The listing builds one solid part. Answer for the finished solid, in the listing's coordinates (mm). A direction names the side the tool comes from. Coordinates: 2 decimals unless noted, no trailing zeros. Order: outer loops, then holes, each group sorted by start corner. A loop starts at its lowest first (then second) coordinate and runs counter-clockwise, first axis right, second up. Notation, with made-up numbers: (-6.5, -7) -> (26.5, -7) arc R9 cw to (26.5, 7) -> close; hole circle Ø1 at (83, 62). An arc over 180 degrees is marked (long way). Return JSON: item names as keys, results as strings.
from build123d import *

# Parameters (mm, degrees)
SKETCH2_W                     = 34
SKETCH2_H                     = 34
BOSS_EXTRUDE_MAIN_DEPTH       = 4.5
SKETCH9_W                     = 14
SKETCH9_H                     = 12.7
CUT_USBC_HOLE_DEPTH           = 5.5
SKETCH10_W                    = 22.5
SKETCH10_H                    = 3.4
CUT_FOURPIN_NOTCH_DEPTH       = 15.7
SKETCH11_R                    = 2
BOSS_EXTRUDE_PEGSPACERS_DEPTH = 2.5
F_2_0MM_HOLES_FOR_PEGS_D      = 1.7
F_2_0MM_HOLES_FOR_PEGS_DEPTH  = 4
F_2_0MM_HOLES_FOR_PEGS_TIP    = 0.510731526
SKETCH15_R                    = 15.4
SKETCH15_R_2                  = 12
CUT_SM1_DEPTH                 = 1
SKETCH18_W                    = 1.4
SKETCH18_H                    = 4.1
CUT_HEXNUTRIGHT_DEPTH         = 1
CUT_HEXNUTRIGHT_DEPTH_BACK    = 6.75
SKETCH19_W                    = 1.4
SKETCH19_H                    = 4.1
CUT_HEXNUTLEFT_DEPTH          = 6.75
SKETCH20_W                    = 18
SKETCH20_H                    = 34
CUT_EXTRUDE2_DEPTH            = 1.5
SKETCH21_W                    = 34
SKETCH21_H                    = 18
CUT_EXTRUDE3_DEPTH            = 1.5
SKETCH22_W                    = 13
SKETCH22_H                    = 10
BOSS_EXTRUDE1_DEPTH           = 10.5
CUT_EXTRUDE4_DEPTH            = 15
SKETCH25_W                    = 2
SKETCH25_H                    = 10
CUT_EXTRUDE5_DEPTH            = 15
SKETCH22_2_W                  = 13
SKETCH22_2_H                  = 10
BOSS_EXTRUDE2_DEPTH           = 1
CUT_EXTRUDE6_DEPTH            = 2
FILLET5_R                     = 3
FILLET4_R                     = 3
FILLET3_R                     = 3
FILLET2_R                     = 3
FILLET7_R                     = 2
FILLET8_R                     = 2
FILLET9_R                     = 1
FILLET10_R                    = 1
FILLET11_R                    = 1
FILLET12_R                    = 1
FILLET13_R                    = 1
FILLET14_R                    = 1
FILLET15_R                    = 1
FILLET16_R                    = 1


with BuildPart() as part:
    # Sketch2 → Boss-Extrude Main (new body)
    with BuildSketch(Plane.XY):
        Rectangle(SKETCH2_W, SKETCH2_H)
    extrude(amount=BOSS_EXTRUDE_MAIN_DEPTH)

    # Sketch9 → Cut-USBc hole (cut, through all)
    with BuildSketch(Plane.XY.offset(4.5)):
        with Locations((0, -8.85)):
            Rectangle(SKETCH9_W, SKETCH9_H)
    extrude(amount=-CUT_USBC_HOLE_DEPTH, mode=Mode.SUBTRACT)

    # Sketch10 → Cut-FourPin Notch (cut)
    with BuildSketch(Plane.XY.offset(4.5)):
        with Locations((1.25, 7.2)):
            Rectangle(SKETCH10_W, SKETCH10_H)
    extrude(amount=-CUT_FOURPIN_NOTCH_DEPTH, mode=Mode.SUBTRACT)

    # Sketch11 → Boss-Extrude_PegSpacers (add)
    with BuildSketch(Plane.XY.offset(4.5)):
        with Locations((-12.25, 12.25)):
            Circle(SKETCH11_R)
        with Locations((12.25, 12.25)):
            Circle(SKETCH11_R)
        with Locations((12.25, -12.25)):
            Circle(SKETCH11_R)
        with Locations((-12.25, -12.25)):
            Circle(SKETCH11_R)
    extrude(amount=BOSS_EXTRUDE_PEGSPACERS_DEPTH)

    # Ø2.0mm Holes for Pegs
    with Locations(Plane(origin=(-12.25, 12.25, 7), x_dir=(1, 0, 0), z_dir=(0, 0, 1))):
        with Locations((0, 0), (24.5, 0), (24.5, -24.5), (0, -24.5)):
            Hole(F_2_0MM_HOLES_FOR_PEGS_D / 2, depth=F_2_0MM_HOLES_FOR_PEGS_DEPTH)
            with Locations((0, 0, -(F_2_0MM_HOLES_FOR_PEGS_DEPTH + F_2_0MM_HOLES_FOR_PEGS_TIP / 2))):  # 118° drill point
                Cone(0, F_2_0MM_HOLES_FOR_PEGS_D / 2, F_2_0MM_HOLES_FOR_PEGS_TIP, mode=Mode.SUBTRACT)

    # Sketch15 → Cut-SM1 (cut)
    with BuildSketch(Plane(origin=(0, 0, 0), x_dir=(-1, 0, 0), z_dir=(0, 0, -1))):
        with Locations((0, -11)):
            Circle(SKETCH15_R)
        with Locations((0, -11)):
            Circle(SKETCH15_R_2, mode=Mode.SUBTRACT)
    extrude(amount=-CUT_SM1_DEPTH, mode=Mode.SUBTRACT)

    # Sketch18 → Cut-HexNutRight (cut, two sides)
    with BuildSketch(Plane(origin=(17, 0, 0), x_dir=(0, 0, -1), z_dir=(1, 0, 0))) as cut_hexnutright_sk:
        with Locations((-3.2, -12.25)):
            Rectangle(SKETCH18_W, SKETCH18_H)
        with Locations((-3.2, 12.25)):
            Rectangle(SKETCH18_W, SKETCH18_H)
    extrude(amount=CUT_HEXNUTRIGHT_DEPTH, mode=Mode.SUBTRACT)
    extrude(cut_hexnutright_sk.sketch, amount=-CUT_HEXNUTRIGHT_DEPTH_BACK, mode=Mode.SUBTRACT)

    # Sketch19 → Cut-HexNutLeft (cut)
    with BuildSketch(Plane.ZY.offset(17)):
        with Locations((3.2, 12.25)):
            Rectangle(SKETCH19_W, SKETCH19_H)
        with Locations((3.2, -12.25)):
            Rectangle(SKETCH19_W, SKETCH19_H)
    extrude(amount=-CUT_HEXNUTLEFT_DEPTH, mode=Mode.SUBTRACT)

    # Sketch20 → Cut-Extrude2 (cut)
    with BuildSketch(Plane.XY.offset(4.5)):
        Rectangle(SKETCH20_W, SKETCH20_H)
    extrude(amount=-CUT_EXTRUDE2_DEPTH, mode=Mode.SUBTRACT)

    # Sketch21 → Cut-Extrude3 (cut)
    with BuildSketch(Plane.XY.offset(4.5)):
        Rectangle(SKETCH21_W, SKETCH21_H)
    extrude(amount=-CUT_EXTRUDE3_DEPTH, mode=Mode.SUBTRACT)

    # Sketch22 → Boss-Extrude1 (add)
    with BuildSketch(Plane.XY):
        with Locations((-21.5, 0)):
            Rectangle(SKETCH22_W, SKETCH22_H)
        with Locations((21.5, 0)):
            Rectangle(SKETCH22_W, SKETCH22_H)
    extrude(amount=BOSS_EXTRUDE1_DEPTH)

    # Sketch24 → Cut-Extrude4 (cut)
    with BuildSketch(Plane(origin=(0, 0, 0), x_dir=(-1, 0, 0), z_dir=(0, 0, -1))):
        with BuildLine():
            Line((21.5, 2.55), (23.5, 2.55))
            ThreePointArc((23.5, 2.55), (26.05, 0), (23.5, -2.55))
            Line((23.5, -2.55), (21.5, -2.55))
            ThreePointArc((21.5, -2.55), (18.95, 0), (21.5, 2.55))
        make_face()
        with BuildLine():
            Line((-21.5, -2.55), (-23.5, -2.55))
            ThreePointArc((-23.5, -2.55), (-26.05, 0), (-23.5, 2.55))
            Line((-23.5, 2.55), (-21.5, 2.55))
            ThreePointArc((-21.5, 2.55), (-18.95, 0), (-21.5, -2.55))
        make_face()
    extrude(amount=-CUT_EXTRUDE4_DEPTH, mode=Mode.SUBTRACT)

    # Sketch25 → Cut-Extrude5 (cut)
    with BuildSketch(Plane.XY.offset(3)):
        with Locations((-16, 0)):
            Rectangle(SKETCH25_W, SKETCH25_H)
        with Locations((16, 0)):
            Rectangle(SKETCH25_W, SKETCH25_H)
    extrude(amount=CUT_EXTRUDE5_DEPTH, mode=Mode.SUBTRACT)

    # Sketch22<2> → Boss-Extrude2 (add)
    with BuildSketch(Plane.XY):
        with Locations((-21.5, 0)):
            Rectangle(SKETCH22_2_W, SKETCH22_2_H)
        with Locations((21.5, 0)):
            Rectangle(SKETCH22_2_W, SKETCH22_2_H)
    extrude(amount=-BOSS_EXTRUDE2_DEPTH)

    # Sketch24<2> → Cut-Extrude6 (cut)
    with BuildSketch(Plane(origin=(0, 0, 0), x_dir=(-1, 0, 0), z_dir=(0, 0, -1))):
        with BuildLine():
            Line((21.5, 2.55), (23.5, 2.55))
            ThreePointArc((23.5, 2.55), (26.05, 0), (23.5, -2.55))
            Line((23.5, -2.55), (21.5, -2.55))
            ThreePointArc((21.5, -2.55), (18.95, 0), (21.5, 2.55))
        make_face()
        with BuildLine():
            Line((-21.5, -2.55), (-23.5, -2.55))
            ThreePointArc((-23.5, -2.55), (-26.05, 0), (-23.5, 2.55))
            Line((-23.5, 2.55), (-21.5, 2.55))
            ThreePointArc((-21.5, 2.55), (-18.95, 0), (-21.5, -2.55))
        make_face()
    extrude(amount=CUT_EXTRUDE6_DEPTH, mode=Mode.SUBTRACT)

    # Fillet5
    fillet5_edges = [part.edges().sort_by_distance(p)[0] for p in [
        (-9, -9, 3.75),
    ]]
    fillet(fillet5_edges, radius=FILLET5_R)

    # Fillet4
    fillet4_edges = [part.edges().sort_by_distance(p)[0] for p in [
        (9, -9, 3.75),
    ]]
    fillet(fillet4_edges, radius=FILLET4_R)

    # Fillet3
    fillet3_edges = [part.edges().sort_by_distance(p)[0] for p in [
        (-9, 9, 3.75),
    ]]
    fillet(fillet3_edges, radius=FILLET3_R)

    # Fillet2
    fillet2_edges = [part.edges().sort_by_distance(p)[0] for p in [
        (9, 9, 3.75),
    ]]
    fillet(fillet2_edges, radius=FILLET2_R)

    # Fillet7
    fillet7_edges = [part.edges().sort_by_distance(p)[0] for p in [
        (-28, 0, -1),
    ]]
    fillet(fillet7_edges, radius=FILLET7_R)

    # Fillet8
    fillet8_edges = [part.edges().sort_by_distance(p)[0] for p in [
        (28, 0, -1),
    ]]
    fillet(fillet8_edges, radius=FILLET8_R)

    # Fillet9
    fillet9_edges = [part.edges().sort_by_distance(p)[0] for p in [
        (-28, 0, 10.5),
    ]]
    fillet(fillet9_edges, radius=FILLET9_R)

    # Fillet10
    fillet10_edges = [part.edges().sort_by_distance(p)[0] for p in [
        (-22, 5, 10.5),
        (-20.5, 5, -1),
        (-27.414213562, 5, -0.414213562),
        (-28, 5, 5.25),
    ]]
    fillet(fillet10_edges, radius=FILLET10_R)

    # Fillet11
    fillet11_edges = [part.edges().sort_by_distance(p)[0] for p in [
        (-17, 5, 6.25),
        (-17, -0.5, 10.5),
    ]]
    fillet(fillet11_edges, radius=FILLET11_R)

    # Fillet12
    fillet12_edges = [part.edges().sort_by_distance(p)[0] for p in [
        (-20.5, -5, -1),
        (-27.414213562, -5, -0.414213562),
        (-28, -5, 5.25),
        (-22.5, -5, 10.5),
        (-17, -5, 6.25),
    ]]
    fillet(fillet12_edges, radius=FILLET12_R)

    # Fillet13
    fillet13_edges = [part.edges().sort_by_distance(p)[0] for p in [
        (28, -5, 5.75),
        (20.5, -5, -1),
        (27.414213562, -5, -0.414213562),
    ]]
    fillet(fillet13_edges, radius=FILLET13_R)

    # Fillet14
    fillet14_edges = [part.edges().sort_by_distance(p)[0] for p in [
        (28, 5, 5.75),
        (20.5, 5, -1),
        (27.414213562, 5, -0.414213562),
    ]]
    fillet(fillet14_edges, radius=FILLET14_R)

    # Fillet15
    fillet15_edges = [part.edges().sort_by_distance(p)[0] for p in [
        (22, -5, 10.5),
        (28, 0, 10.5),
        (22, 5, 10.5),
    ]]
    fillet(fillet15_edges, radius=FILLET15_R)

    # Fillet16
    fillet16_edges = [part.edges().sort_by_distance(p)[0] for p in [
        (17, 5, 6.25),
        (17, 0, 10.5),
        (17, -5, 6.25),
    ]]
    fillet(fillet16_edges, radius=FILLET16_R)


solid = part.part
1. For faces 4 (the face through (-17.301, -0.056, 10.215)), 5 (the face through (-14, 12, 3.9)), 6 (the face through (0, -16, 0)), 7 (the face through (10.25, 12, 3)), 8 (the face through (12.5, 7, 2)), determine the directions among +Z, -Z, +X, -X, +Y, -Y from which every point of the face is accessible in a straight line to the end or side of a thin tool.
Answer block:
{"face 4": "+Z, +Y, -Y", "face 5": "-X", "face 6": "-Z, +Y, -Y", "face 7": "+X", "face 8": "+Z, -Z"}
2. The part is cut by section A-A on x = 0. Give the vertices of the cut face in (y, z).
Answer block:
{"outline": "(-17, 0) -> (-15.2, 0) -> (-15.2, 3) -> (-17, 3) -> close; (-2.5, 0) -> (1, 0) -> (1, 1) -> (4.4, 1) -> (4.4, 0) -> (5.5, 0) -> (5.5, 3) -> (-2.5, 3) -> close; (8.9, 0) -> (17, 0) -> (17, 3) -> (8.9, 3) -> close"}
3. Each of these flat-tipped pins is pushed along its axis until it touches: pin 1 Ø0.7 at (y, z) = (-11.5, 3) entering from +X; pin 2 Ø1.1 at (y, z) = (-1, -0.5) entering from -X; pin 3 Ø2 at (x, y) = (12.5, 13) entering from +Z; pin 4 Ø1.5 at (x, z) = (8.5, 9) entering from +Y. Where does it stop, or does it pass through?
Answer block:
{"pin 1": "stops at x = 10.25", "pin 2": "stops at x = -27.76", "pin 3": "stops at z = 7", "pin 4": "passes through"}
4. The part is cut by section B-B on z = 6. Give the number of separate pieces and of enclosed holes in the cut face, and give its area (3 significant figures).
Answer block:
{"separate pieces": "6", "enclosed holes": "6", "area": "198 mm2"}
5. Consider line 1 (Y direction, x = 12.25, z = 5.9); line 2 (X direction, y = -3, z = 7.5); line 3 (Y direction, x = -11, z = 3.5). Determine where each line is inside the solid, lowest interval first. Write a range as from..to.
Answer block:
{"line 1": "y = -14.25..-13.1, -11.4..-10.25, 10.25..11.4, 13.1..14.25", "line 2": "x = -28..-17, 17..28", "line 3": "y = -17..-14.3, -10.2..-9.17, 9.17..10.2, 14.3..17"}
6. The part is cut by section C-C on y = 15. Give the vertices of the cut face in (x, z).
Answer block:
{"outline": "(-17, 0) -> (17, 0) -> (17, 4.5) -> (9, 4.5) -> (9, 3) -> (-9, 3) -> (-9, 4.5) -> (-17, 4.5) -> close"}
7. Determine the mould class of faces 1 (the face through (17, 0, 6)), 2 (the face through (17, -11, 2)), 3 (the face through (27.699, -4.715, 5.31)) for opening direction Y: pulls with the +Y half, pulls with the -Y half, needs draft (parallel to the pull), parting line crosses it, or undercut.
Answer block:
{"face 1": "undercut", "face 2": "needs draft", "face 3": "pulls with the -Y half"}
